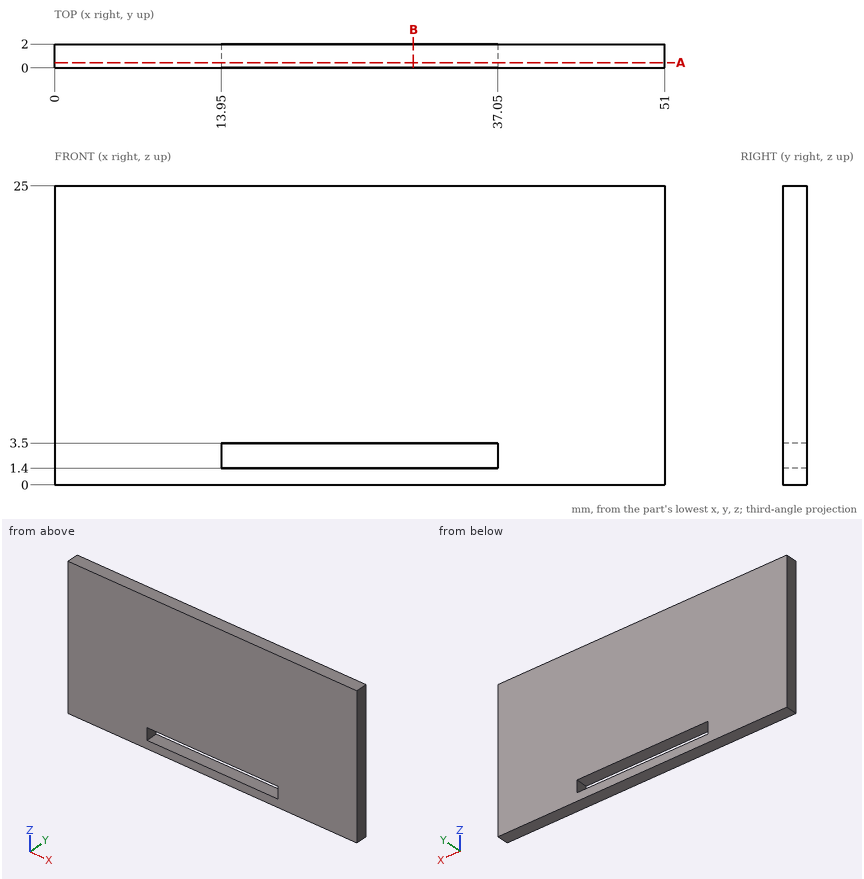
Geometry check sheet. Reference: drawing and pictorial views, mm from the part's lowest x, y, z. Coordinates: 2 decimals unless noted, no trailing zeros. Order: outer loops, then holes, each group sorted by start corner. A loop starts at its lowest first (then second) coordinate and runs counter-clockwise, first axis right, second up.
Item 1: Section check B-B, the plane x = 30. Enter the section's corners in (y, z), then the cut area to 3 significant figures.
Filled in:
outline: (0, 0) - (2, 0) - (2, 1.4) - (0, 1.4) - close; (0, 3.5) - (2, 3.5) - (2, 25) - (0, 25) - close
area: 45.8 mm2
Item 2: Section check A-A, the plane y = 0.45. Enter the section's corners in (x, z).
Filled in:
outline: (0, 0) - (51, 0) - (51, 25) - (0, 25) - close; hole (13.95, 1.4) - (37.05, 1.4) - (37.05, 3.5) - (13.95, 3.5) - close
Item 3: Material ranges on L1, parallel to Z at x = 35.5, y = 0.4; L2, parallel to X at y = 0.75, z = 3.25, recorded low to high.
Filled in:
L1: z = 0 to 1.4, 3.5 to 25
L2: x = 0 to 13.95, 37.05 to 51
